Here's how the part is built. I have some questions about the finished solid (model axes, mm). Face numbers are marked on the shaded views. A direction names the side the tool comes from. Round coordinates to 2 decimals unless told otherwise and drop trailing zeros. Write each loop counter-clockwise with the first axis right and the second up, starting at its lowest first coordinate (ties: lowest second). Pieces come first, ordered by that corner, then holes. Notation, with made-up numbers: (83, -15) - (107, -15) arc R23 ccw to (107, -4) - close; hole circle Ø2 at (21.5, 41). An arc over 180 degrees is marked (long way). Write item = value, one per line. Start each with the question number.
Item 1: Thinking about a two-plate mould opening in Z: for the marked faces 1, 2, 3 and 4, which applies, pulls with the +Z half, pulls with the -Z half, needs draft (parallel to the pull), parting line crosses it, or undercut?
Item 2: If we section it at C-C (z = -19.05): Give the number of separate pieces and of enclosed holes in the cut face, and give its area (3 significant figures).
Item 3: For P1, Ø1, axis at y = 30.5, z = 11.5, coming from the -X side; P2, Ø8, axis at x = 60, z = 4, coming from the +Y side, each with a flat end and sliding along its axis, tell me the tip position at first contact or that it passes through.
Item 4: If we section it at B-B (x = -9): Please give me the cut outline in (y, z), and give its area (3 significant figures).
Item 5: Which directions (+Z, -Z, +X, -X, +Y, -Y) give clear straight access to the entire face, cutting with the end or side of a thin tool? Please do the marked faces 5, 6 and 7.
Item 6: If we section it at A-A (z = 19.05): Please give me the cut outline in (x, y), and give its area (3 significant figures).
Item 7: If I drill on line 1 along X through (y, z) = (39.5, -32); line 2 along X through (y, z) = (4, -36.5); line 3 along Z through (x, y) = (-19, 11), over which ranges is the centre line in solid material (lowest first)? Write a range as [from, to].
```python
from build123d import *

# Parameters (mm, degrees)
SKETCH1_W           = 165.1
SKETCH1_H           = 101.6
SKETCH1_R           = 2.54
SKETCH1_W_2         = 133.35
SKETCH1_H_2         = 88.9
SKETCH1_W_3         = 25.4
MOUNTING_BASE_DEPTH = 6.35
SKETCH2_W           = 165.1
SKETCH2_H           = 101.6
SKETCH2_W_2         = 6.35
SKETCH2_H_2         = 88.9
WALLS_DEPTH         = 38.1
SKETCH3_R           = 14.2875
BEARING_HOLES_DEPTH = 38.1
SKETCH4_R           = 7.62
SHAFT_HOLES_DEPTH   = 38.1
SKETCH5_R           = 2.54
MOD_HOLES_DEPTH     = 139.249285712
OUTSIDE_VERTICES_R  = 12.7
INSIDE_VERTICES_R   = 6.35


with BuildPart() as part:
    # Sketch1 → Mounting Base (new body)
    # profile 1 of 3: a face of its own
    with BuildSketch(Plane(origin=(0, 0, 0), x_dir=(1, 0, 0), z_dir=(0, 1, 0))):
        Rectangle(SKETCH1_W, SKETCH1_H)
        with Locations(Location((66.675, 9.525, 0), (0, 0, 270))):
            Circle(SKETCH1_R, mode=Mode.SUBTRACT)
        with Locations(Location((66.675, 28.575, 0), (0, 0, 270))):
            Circle(SKETCH1_R, mode=Mode.SUBTRACT)
        with Locations((-9.525, 0)):
            Rectangle(SKETCH1_W_2, SKETCH1_H_2, mode=Mode.SUBTRACT)
    # profile 2 of 3: a face of its own
    with BuildSketch(Plane(origin=(0, 0, 0), x_dir=(1, 0, 0), z_dir=(0, 1, 0))):
        with Locations((-44.45, 0)):
            Rectangle(SKETCH1_W_3, SKETCH1_H_2)
        with Locations(Location((-41.275, -28.575, 0), (0, 0, 270))):
            Circle(SKETCH1_R, mode=Mode.SUBTRACT)
        with Locations(Location((-41.275, -9.525, 0), (0, 0, 270))):
            Circle(SKETCH1_R, mode=Mode.SUBTRACT)
    # profile 3 of 3: a face of its own
    with BuildSketch(Plane(origin=(0, 0, 0), x_dir=(1, 0, 0), z_dir=(0, 1, 0))):
        with Locations((12.7, 0)):
            Rectangle(SKETCH1_W_3, SKETCH1_H_2)
        with Locations(Location((5.715, -28.575, 0), (0, 0, 270))):
            Circle(SKETCH1_R, mode=Mode.SUBTRACT)
        with Locations(Location((5.715, -9.525, 0), (0, 0, 270))):
            Circle(SKETCH1_R, mode=Mode.SUBTRACT)
        with Locations(Location((19.685, 9.525, 0), (0, 0, 270))):
            Circle(SKETCH1_R, mode=Mode.SUBTRACT)
        with Locations(Location((19.685, 28.575, 0), (0, 0, 270))):
            Circle(SKETCH1_R, mode=Mode.SUBTRACT)
    extrude(amount=MOUNTING_BASE_DEPTH)

    # Sketch2 → Walls (add)
    # profile 1 of 2: a face of its own
    with BuildSketch(Plane(origin=(0, 6.35, 0), x_dir=(1, 0, 0), z_dir=(0, 1, 0))):
        Rectangle(SKETCH2_W, SKETCH2_H)
        Polygon((-57.15, -44.45), (-76.2, -44.45), (-76.2, 44.45), (-57.15, 44.45), (-50.8, 44.45), (-31.75, 44.45), (0, 44.45), (25.4, 44.45), (57.15, 44.45), (76.2, 44.45), (76.2, -44.45), (57.15, -44.45), (25.4, -44.45), (0, -44.45), (-31.75, -44.45), (-50.8, -44.45), align=None, mode=Mode.SUBTRACT)
    # profile 2 of 2: a face of its own
    with BuildSketch(Plane(origin=(0, 6.35, 0), x_dir=(1, 0, 0), z_dir=(0, 1, 0))):
        with Locations((-53.975, 0)):
            Rectangle(SKETCH2_W_2, SKETCH2_H_2)
    extrude(amount=WALLS_DEPTH)

    # Sketch3 → Bearing Holes (cut)
    with BuildSketch(Plane.ZY.offset(82.55)):
        with Locations((-19.05, 25.4)):
            Circle(SKETCH3_R)
        with Locations((19.05, 25.4)):
            Circle(SKETCH3_R)
    extrude(amount=-BEARING_HOLES_DEPTH, mode=Mode.SUBTRACT)

    # Sketch4 → Shaft Holes (cut)
    with BuildSketch(Plane(origin=(82.55, 0, 0), x_dir=(0, 0, -1), z_dir=(1, 0, 0))):
        with Locations((19.05, 25.4)):
            Circle(SKETCH4_R)
    extrude(amount=-SHAFT_HOLES_DEPTH, mode=Mode.SUBTRACT)

    # Sketch5 → Mod Holes (cut, through all)
    with BuildSketch(Plane(origin=(0, 0, -50.8), x_dir=(-1, 0, 0), z_dir=(0, 0, -1))):
        with Locations((-41.275, 34.29)):
            Circle(SKETCH5_R)
        with Locations((-41.275, 12.065)):
            Circle(SKETCH5_R)
        with Locations((41.275, 34.29)):
            Circle(SKETCH5_R)
        with Locations((41.275, 12.065)):
            Circle(SKETCH5_R)
        with Locations((0, 34.29)):
            Circle(SKETCH5_R)
        with Locations((0, 12.065)):
            Circle(SKETCH5_R)
    extrude(amount=-MOD_HOLES_DEPTH, mode=Mode.SUBTRACT)

    # Outside Vertices
    outside_vertices_edges = [part.edges().sort_by_distance(p)[0] for p in [
        (-82.55, 22.225, 50.8),
        (-82.55, 22.225, -50.8),
        (82.55, 22.225, -50.8),
        (82.55, 22.225, 50.8),
    ]]
    fillet(outside_vertices_edges, radius=OUTSIDE_VERTICES_R)

    # Inside Vertices
    inside_vertices_edges = [part.edges().sort_by_distance(p)[0] for p in [
        (-76.2, 22.225, 44.45),
        (-76.2, 22.225, -44.45),
        (76.2, 25.4, 44.45),
        (76.2, 25.4, -44.45),
        (-50.8, 25.4, -44.45),
        (-50.8, 25.4, 44.45),
        (-57.15, 22.225, 44.45),
        (-57.15, 22.225, -44.45),
    ]]
    fillet(inside_vertices_edges, radius=INSIDE_VERTICES_R)


solid = part.part
```
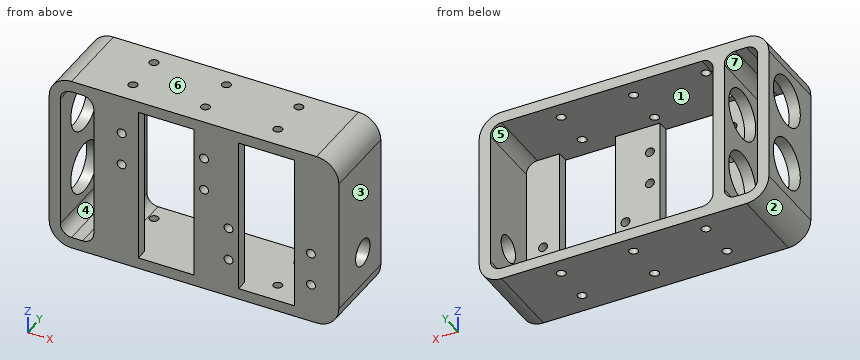
Reply:
q1.face_1 = undercut
q1.face_2 = pulls with the -Z half
q1.face_3 = needs draft
q1.face_4 = undercut
q2.separate_pieces = 7
q2.enclosed_holes = 0
q2.area = 790 mm2
q3.P1 = 76.2
q3.P2 = 6.35
q4.outline = (0, -50.8) - (44.45, -50.8) - (44.45, -44.45) - (0, -44.45) - close; (0, 44.45) - (44.45, 44.45) - (44.45, 50.8) - (0, 50.8) - close
q4.area = 565 mm2
q5.face_5 = +Y
q5.face_6 = +Z, +X, -X, +Y, -Y
q5.face_7 = +Y, -Y
q6.outline = (-82.55, 0) - (-76.2, 0) - (-76.2, 11.11) - (-82.55, 11.11) - close; (-82.55, 39.69) - (-76.2, 39.69) - (-76.2, 44.45) - (-82.55, 44.45) - close; (-57.15, 0) - (-31.75, 0) - (-31.75, 6.35) - (-50.8, 6.35) - (-50.8, 11.11) - (-57.15, 11.11) - close; (-57.15, 39.69) - (-50.8, 39.69) - (-50.8, 44.45) - (-57.15, 44.45) - close; (0, 0) - (25.4, 0) - (25.4, 6.35) - (0, 6.35) - close; (57.15, 0) - (82.55, 0) - (82.55, 44.45) - (76.2, 44.45) - (76.2, 6.35) - (57.15, 6.35) - close
q6.area = 887 mm2
q7.line_1 = [-82.55, -76.2], [-57.15, -50.8], [76.2, 82.55]
q7.line_2 = [-82.55, -76.2], [-57.15, -31.75], [0, 25.4], [57.15, 82.55]
q7.line_3 = [-50.8, -44.45], [44.45, 50.8]
